Design review of the part built by this model. Coordinates are the model's own, in mm. Face numbers are marked on the shaded views. Round coordinates to 2 decimals unless told otherwise and drop trailing zeros. Order: outer loops, then holes, each group sorted by start corner. A loop starts at its lowest first (then second) coordinate and runs counter-clockwise, first axis right, second up. Notation, with made-up numbers: (61.25, 17.25) - (67.25, 17.25) arc R23 ccw to (67.25, 50.25) - close; hole circle Ø8 at (63.5, -11.75). An arc over 180 degrees is marked (long way). Write item = value, one per line.
from build123d import *

# Parameters (mm, degrees)
SKETCH_1_R      = 15
EXTRUDE_1_DEPTH = 1
SKETCH_2_R      = 13.7
SKETCH_2_R_2    = 12
EXTRUDE_2_DEPTH = 9
FILLET_1_R      = 0.2


with BuildPart() as part:
    # 草图1 → 凸台-拉伸1 (new body)
    with BuildSketch(Plane(origin=(0, 0, 0), x_dir=(1, 0, 0), z_dir=(0, 1, 0))):
        with Locations(Location((0, 0, 0), (0, 0, 270))):
            Circle(SKETCH_1_R)
    extrude(amount=EXTRUDE_1_DEPTH)

    # 草图2 → 凸台-拉伸2 (add)
    with BuildSketch(Plane(origin=(0, 1, 0), x_dir=(1, 0, 0), z_dir=(0, 1, 0))):
        with Locations(Location((0, 0, 0), (0, 0, 270))):
            Circle(SKETCH_2_R)
        with Locations(Location((0, 0, 0), (0, 0, 270))):
            Circle(SKETCH_2_R_2, mode=Mode.SUBTRACT)
    extrude(amount=EXTRUDE_2_DEPTH)

    # 圆角1
    fillet_1_edges = [part.edges().sort_by_distance(p)[0] for p in [
        (0, 0, -15),
        (0, 1, -15),
        (0, 10, -13.7),
        (0, 10, -12),
    ]]
    fillet(fillet_1_edges, radius=FILLET_1_R)


solid = part.part
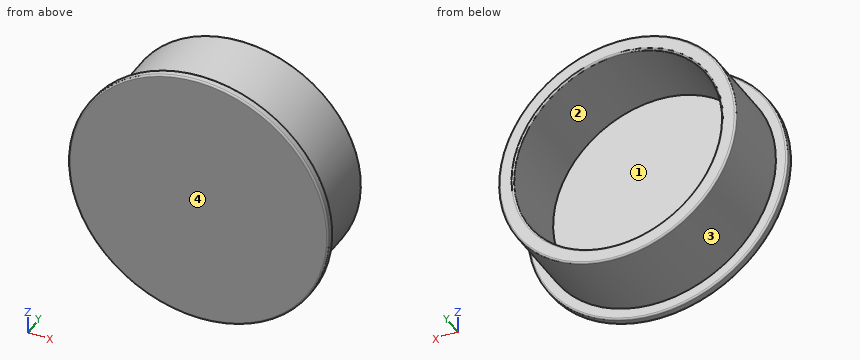
Item 1: Take a section at B-B, the plane z = 0. State the section outline as (x, y) points, and give its area (3 significant figures).
Data:
outline = (-15, 0.2) arc R0.2 ccw to (-14.8, 0) - (14.8, 0) arc R0.2 ccw to (15, 0.2) - (15, 0.8) arc R0.2 ccw to (14.8, 1) - (13.7, 1) - (13.7, 9.8) arc R0.2 ccw to (13.5, 10) - (12.2, 10) arc R0.2 ccw to (12, 9.8) - (12, 1) - (-12, 1) - (-12, 9.8) arc R0.2 ccw to (-12.2, 10) - (-13.5, 10) arc R0.2 ccw to (-13.7, 9.8) - (-13.7, 1) - (-14.8, 1) arc R0.2 ccw to (-15, 0.8) - close
area = 60.5 mm2
Item 2: Take a section at C-C, the plane y = 5.75. State the section outline as (x, z) points, and give its area (3 significant figures).
Data:
outline = circle Ø27.4 at (0, 0); hole circle Ø24 at (0, 0)
area = 137 mm2
Item 3: Insertion check: P1, Ø6, axis at y = 2.5, z = -8.5, coming from the -X side; P2, Ø4, axis at x = 4.5, z = -2, coming from the +Y side; P3, Ø1.5, axis at x = 0, y = 8.5, coming from the -Z side; P4, Ø6, axis at x = 9, z = -6.5, coming from the -Y side. Each pin has a flat end and moves straight along its axis. Give the tip position at first contact, or say it passes through.
Data:
P1 = -13.74
P2 = 1
P3 = -13.7
P4 = 0
Item 4: The part is to be moulded in two halves that separate along X. For the marked faces 1, 2, 3 and 4, say which applies: +X half, -X half, draft (parallel to the pull), parting line (faces both ways), or undercut.
Data:
face_1 = undercut
face_2 = undercut
face_3 = parting line
face_4 = draft
Item 5: For line 1 along X through (y, z) = (3.25, 0); line 2 along Y through (x, z) = (-2, -6); line 3 along X through (y, z) = (8.5, -2.25), list the stretches that pass through material, from the lowest coordinate up. Write a range as [from, to].
Data:
line_1 = [-13.7, -12], [12, 13.7]
line_2 = [0, 1]
line_3 = [-13.51, -11.79], [11.79, 13.51]
Item 6: Take a section at A-A, the plane x = 0. State the section outline as (y, z) points, and give its area (3 significant figures).
Data:
outline = (0, -14.8) arc R0.2 ccw to (0.2, -15) - (0.8, -15) arc R0.2 ccw to (1, -14.8) - (1, -13.7) - (9.8, -13.7) arc R0.2 ccw to (10, -13.5) - (10, -12.2) arc R0.2 ccw to (9.8, -12) - (1, -12) - (1, 12) - (9.8, 12) arc R0.2 ccw to (10, 12.2) - (10, 13.5) arc R0.2 ccw to (9.8, 13.7) - (1, 13.7) - (1, 14.8) arc R0.2 ccw to (0.8, 15) - (0.2, 15) arc R0.2 ccw to (0, 14.8) - close
area = 60.5 mm2
